```python
from build123d import *

# Parameters (mm, degrees)
SKETCH1_R           = 63.5
SKETCH1_R_2         = 1.5875
BOSS_EXTRUDE3_DEPTH = 6.35
SKETCH1_7_R         = 76.2
SKETCH1_7_R_2       = 63.5
SKETCH1_7_R_3       = 1.5875
BOSS_EXTRUDE4_DEPTH = 3.175


with BuildPart() as part:
    # Sketch1 → Boss-Extrude3 (new body)
    with BuildSketch(Plane(origin=(0, 0, 0), x_dir=(1, 0, 0), z_dir=(0, 1, 0))):
        with Locations(Location((0, 0, 0), (0, 0, 270))):
            Circle(SKETCH1_R)
        with BuildLine():
            Line((-50.652943399, -3.175), (-36.686174209, -3.175))
            Line((-36.686174209, -3.175), (-46.540477324, -20.243153668))
            ThreePointArc((-46.540477324, -20.243153668), (-49.340355951, -11.88825364), (-50.652943399, -3.175))
        make_face(mode=Mode.SUBTRACT)
        with Locations(Location((-20.955, -37.4523, 0), (0, 0, 270))):
            Circle(SKETCH1_R_2, mode=Mode.SUBTRACT)
        with BuildLine():
            Line((-33.02, -9.525), (-33.02, -38.5419369))
            ThreePointArc((-33.02, -38.5419369), (-38.476065533, -33.096732181), (-43.04456039, -26.888047918))
            Line((-43.04456039, -26.888047918), (-33.02, -9.525))
        make_face(mode=Mode.SUBTRACT)
        with Locations(Location((20.955, -37.4523, 0), (0, 0, 270))):
            Circle(SKETCH1_R_2, mode=Mode.SUBTRACT)
        with BuildLine():
            ThreePointArc((43.04456039, -26.888047918), (38.476065533, -33.096732181), (33.02, -38.5419369))
            Line((33.02, -38.5419369), (33.02, -9.525))
            Line((33.02, -9.525), (43.04456039, -26.888047918))
        make_face(mode=Mode.SUBTRACT)
        with BuildLine():
            Line((46.540477324, -20.243153668), (36.686174209, -3.175))
            Line((36.686174209, -3.175), (50.652943399, -3.175))
            ThreePointArc((50.652943399, -3.175), (49.340355951, -11.88825364), (46.540477324, -20.243153668))
        make_face(mode=Mode.SUBTRACT)
        with BuildLine():
            Line((-46.540477324, 20.243153668), (-36.686174209, 3.175))
            Line((-36.686174209, 3.175), (-50.652943399, 3.175))
            ThreePointArc((-50.652943399, 3.175), (-49.340355951, 11.88825364), (-46.540477324, 20.243153668))
        make_face(mode=Mode.SUBTRACT)
        with BuildLine():
            Line((-33.02, 38.5419369), (-33.02, 9.525))
            Line((-33.02, 9.525), (-43.04456039, 26.888047918))
            ThreePointArc((-43.04456039, 26.888047918), (-38.476065533, 33.096732181), (-33.02, 38.5419369))
        make_face(mode=Mode.SUBTRACT)
        with Locations(Location((-24.13, 28.5496, 0), (0, 0, 270))):
            Circle(SKETCH1_R_2, mode=Mode.SUBTRACT)
        Polygon((17.145, -43.18), (-17.145, -43.18), (-17.145, -33.6423), (-26.67, -33.6423), (-26.67, 24.7396), (-20.955, 24.7396), (-20.955, 31.2547), (-26.67, 31.2547), (-26.67, 43.18), (26.67, 43.18), (26.67, 31.2547), (20.955, 31.2547), (20.955, 24.7396), (26.67, 24.7396), (26.67, -33.6423), (17.145, -33.6423), align=None, mode=Mode.SUBTRACT)
        with Locations(Location((24.13, 28.5496, 0), (0, 0, 270))):
            Circle(SKETCH1_R_2, mode=Mode.SUBTRACT)
        with BuildLine():
            Line((43.04456039, 26.888047918), (33.02, 9.525))
            Line((33.02, 9.525), (33.02, 38.5419369))
            ThreePointArc((33.02, 38.5419369), (38.476065533, 33.096732181), (43.04456039, 26.888047918))
        make_face(mode=Mode.SUBTRACT)
        with BuildLine():
            Line((50.652943399, 3.175), (36.686174209, 3.175))
            Line((36.686174209, 3.175), (46.540477324, 20.243153668))
            ThreePointArc((46.540477324, 20.243153668), (49.340355951, 11.88825364), (50.652943399, 3.175))
        make_face(mode=Mode.SUBTRACT)
    extrude(amount=BOSS_EXTRUDE3_DEPTH)

    # Sketch1_7 → Boss-Extrude4 (add)
    with BuildSketch(Plane(origin=(0, 0, 0), x_dir=(1, 0, 0), z_dir=(0, 1, 0))):
        with Locations(Location((0, 0, 0), (0, 0, 270))):
            Circle(SKETCH1_7_R)
        with Locations(Location((0, 0, 0), (0, 0, 270))):
            Circle(SKETCH1_7_R_2, mode=Mode.SUBTRACT)
        with Locations(Location((-18.0785103, 67.469918966, 0), (0, 0, 270))):
            Circle(SKETCH1_7_R_3, mode=Mode.SUBTRACT)
        with Locations(Location((-34.925, 60.491874454, 0), (0, 0, 270))):
            Circle(SKETCH1_7_R_3, mode=Mode.SUBTRACT)
        with Locations(Location((-49.391408666, 49.391408666, 0), (0, 0, 270))):
            Circle(SKETCH1_7_R_3, mode=Mode.SUBTRACT)
        with Locations(Location((-60.491874454, 34.925, 0), (0, 0, 270))):
            Circle(SKETCH1_7_R_3, mode=Mode.SUBTRACT)
        with Locations(Location((-67.469918966, 18.0785103, 0), (0, 0, 270))):
            Circle(SKETCH1_7_R_3, mode=Mode.SUBTRACT)
        with Locations(Location((-69.85, 0, 0), (0, 0, 270))):
            Circle(SKETCH1_7_R_3, mode=Mode.SUBTRACT)
        with Locations(Location((-67.469918966, -18.0785103, 0), (0, 0, 270))):
            Circle(SKETCH1_7_R_3, mode=Mode.SUBTRACT)
        with Locations(Location((-60.491874454, -34.925, 0), (0, 0, 270))):
            Circle(SKETCH1_7_R_3, mode=Mode.SUBTRACT)
        with Locations(Location((-49.391408666, -49.391408666, 0), (0, 0, 270))):
            Circle(SKETCH1_7_R_3, mode=Mode.SUBTRACT)
        with Locations(Location((-34.925, -60.491874454, 0), (0, 0, 270))):
            Circle(SKETCH1_7_R_3, mode=Mode.SUBTRACT)
        with Locations(Location((-18.0785103, -67.469918966, 0), (0, 0, 270))):
            Circle(SKETCH1_7_R_3, mode=Mode.SUBTRACT)
        with Locations(Location((0, -69.85, 0), (0, 0, 270))):
            Circle(SKETCH1_7_R_3, mode=Mode.SUBTRACT)
        with Locations(Location((18.0785103, -67.469918966, 0), (0, 0, 270))):
            Circle(SKETCH1_7_R_3, mode=Mode.SUBTRACT)
        with Locations(Location((34.925, -60.491874454, 0), (0, 0, 270))):
            Circle(SKETCH1_7_R_3, mode=Mode.SUBTRACT)
        with Locations(Location((49.391408666, -49.391408666, 0), (0, 0, 270))):
            Circle(SKETCH1_7_R_3, mode=Mode.SUBTRACT)
        with Locations(Location((60.491874454, -34.925, 0), (0, 0, 270))):
            Circle(SKETCH1_7_R_3, mode=Mode.SUBTRACT)
        with Locations(Location((67.469918966, -18.0785103, 0), (0, 0, 270))):
            Circle(SKETCH1_7_R_3, mode=Mode.SUBTRACT)
        with Locations(Location((69.85, 0, 0), (0, 0, 270))):
            Circle(SKETCH1_7_R_3, mode=Mode.SUBTRACT)
        with Locations(Location((67.469918966, 18.0785103, 0), (0, 0, 270))):
            Circle(SKETCH1_7_R_3, mode=Mode.SUBTRACT)
        with Locations(Location((60.491874454, 34.925, 0), (0, 0, 270))):
            Circle(SKETCH1_7_R_3, mode=Mode.SUBTRACT)
        with Locations(Location((49.391408666, 49.391408666, 0), (0, 0, 270))):
            Circle(SKETCH1_7_R_3, mode=Mode.SUBTRACT)
        with Locations(Location((34.925, 60.491874454, 0), (0, 0, 270))):
            Circle(SKETCH1_7_R_3, mode=Mode.SUBTRACT)
        with Locations(Location((0, 69.85, 0), (0, 0, 270))):
            Circle(SKETCH1_7_R_3, mode=Mode.SUBTRACT)
        with Locations(Location((18.0785103, 67.469918966, 0), (0, 0, 270))):
            Circle(SKETCH1_7_R_3, mode=Mode.SUBTRACT)
    extrude(amount=BOSS_EXTRUDE4_DEPTH)


solid = part.part
```
The listing builds one solid part. Answer for the finished solid, in the listing's coordinates (mm). A direction names the side the tool comes from. Coordinates: 2 decimals unless noted, no trailing zeros. Write each loop counter-clockwise with the first axis right and the second up, starting at its lowest first coordinate (ties: lowest second). Pieces come first, ordered by that corner, then holes. Notation, with made-up numbers: (-23, 62.25) -> (4, 62.25) arc R15 cw to (4, 79.25) -> close; hole circle Ø5 at (41.5, -24). An arc over 180 degrees is marked (long way). Write each question's results on one line, items separated by ' | '. Start each with the question number.
1) Straight lines are drawn through the part: probe 1 along X at (y, z) = (1.25, 14); probe 2 along Z at (x, y) = (-24, 2.75); probe 3 along Z at (x, y) = (19.5, 3.5). For each, find the intervals that lie inside material, in ascending order.
2) For a pull along X with two mould halves and no side action, classify faces 1 (the flat face through (-33, 0, -1)), 2 (the flat face through (0, 3, -43.18)), 3 (the cylindrical face through (-61.99, 4.74, -13.77)) as +X half, -X half, draft (parallel to the pull), parting line (faces both ways), or undercut.
3) A tool of negligible diameter and unlimited length cuts with its end or side. For faces 4 (the flat face through (-33.02, 3, 24)), 5 (the flat face through (-27, 6.35, -1)), 6 (the flat face through (-45, 3.175, -46)), from which of +Z, -Z, +X, -X, +Y, -Y can it reach the whole face along a straight path? Write none if from no direction.
4) A cutting plane is placed at B-B (y = 5.25). Count the separate pieces of the cut face and the enclosed holes in it, then the cut area to 3 significant figures.
5) A cutting plane is placed at D-D (x = -54). Determine the outline of the cut face in (y, z) (3 decimals).
6) Flat-ended cylindrical pins translate along their axes: pin 1 Ø4 at (x, z) = (34.92, -60.49) entering from +Y (3 decimals); pin 2 Ø1.9 at (x, y) = (20, 4) entering from -Z (3 decimals); pin 3 Ø1 at (x, y) = (-39.5, 5) entering from +Z. Find the tip coordinate at first contact, or state that the pin passes through.
7) A cutting plane is placed at C-C (z = -41). Determine the outline of the cut face in (x, y) (3 decimals).
8) A cutting plane is placed at A-A (z = 13). Determine the outline of the cut face in (x, y) (3 decimals).
Values follow:
1) probe 1: -74.9 to -48.78, -42.94 to -35.6, -33.02 to -26.67, 26.67 to 33.02, 35.6 to 42.94, 48.78 to 74.9 | probe 2: -72.32 to -43.18, -31.25 to -30.13, -26.97 to -24.74, 33.64 to 72.32 | probe 3: -60.43 to -43.18, 33.64 to 36.82, 38.09 to 60.43
2) face 1: draft | face 2: undercut | face 3: parting line
3) face 4: +Y, -Y | face 5: +Z, -Z, +X, -X, +Y | face 6: +Y
4) separate pieces: 1 | enclosed holes: 13 | area: 7,170 mm²
5) outline: (0, -53.763) -> (3.175, -53.763) -> (3.175, -33.41) -> (6.35, -33.41) -> (6.35, 33.41) -> (3.175, 33.41) -> (3.175, 53.763) -> (0, 53.763) -> close
6) pin 1: y = 3.175 | pin 2: z = -73.655 | pin 3: z = 50.11
7) outline: (-64.23, 0) -> (-26.67, 0) -> (-26.67, 6.35) -> (-48.49, 6.35) -> (-48.49, 3.175) -> (-64.23, 3.175) -> close; (26.67, 0) -> (64.23, 0) -> (64.23, 3.175) -> (48.49, 3.175) -> (48.49, 6.35) -> (26.67, 6.35) -> close
8) outline: (-75.083, 0) -> (-49.059, 0) -> (-49.059, 6.35) -> (-62.155, 6.35) -> (-62.155, 3.175) -> (-75.083, 3.175) -> close; (-42.359, 0) -> (-35.026, 0) -> (-35.026, 6.35) -> (-42.359, 6.35) -> close; (-33.02, 0) -> (-26.67, 0) -> (-26.67, 6.35) -> (-33.02, 6.35) -> close; (26.67, 0) -> (33.02, 0) -> (33.02, 6.35) -> (26.67, 6.35) -> close; (35.026, 0) -> (42.359, 0) -> (42.359, 6.35) -> (35.026, 6.35) -> close; (49.059, 0) -> (75.083, 0) -> (75.083, 3.175) -> (62.155, 3.175) -> (62.155, 6.35) -> (49.059, 6.35) -> close
